For this review, take the finished solid that the model builds, in its own axes (mm). Face numbers are marked on the shaded views. A direction names the side the tool comes from. Coordinates: 2 decimals unless noted, no trailing zeros. Loops run counter-clockwise (first coordinate to the right, second up) from the corner with the lowest first, then second, coordinate; pieces in that order, holes last. Notation, with made-up numbers: (-12, 45.5) -> (13, 45.5) arc R26 ccw to (13, 68.5) -> close; hole circle Ø7 at (20, -38.75). An arc over 180 degrees is marked (long way). Use a Markdown table: item, result.
from build123d import *

# Parameters (mm, degrees)
EXTRUDE_1_DEPTH     = 10
SKETCH_2_R          = 6.5
CUT_EXTRUDE_1_DEPTH = 10
CUT_EXTRUDE_2_DEPTH = 10
FILLET_1_R          = 1
SKETCH_4_R          = 6.5
CUT_EXTRUDE_3_DEPTH = 10


with BuildPart() as part:
    # 草图1 → 凸台-拉伸1 (new body)
    with BuildSketch(Plane.XY):
        with BuildLine():
            Line((200.1875, 14.998828079), (0.21875, 17.498632759))
            ThreePointArc((0.21875, 17.498632759), (-17.5, 0), (0.21875, -17.498632759))
            Line((0.21875, -17.498632759), (200.1875, -14.998828079))
            ThreePointArc((200.1875, -14.998828079), (215, 0), (200.1875, 14.998828079))
        make_face()
    extrude(amount=EXTRUDE_1_DEPTH)

    # 草图2 → 切除-拉伸1 (cut)
    with BuildSketch(Plane.XY.offset(10)):
        Circle(SKETCH_2_R)
    extrude(amount=-CUT_EXTRUDE_1_DEPTH, mode=Mode.SUBTRACT)

    # 草图3 → 切除-拉伸2 (cut)
    with BuildSketch(Plane.XY.offset(10)):
        Polygon((24.289001935, 12.19734043), (85.658139631, 11.430166271), (16.937408094, -6.979422532), align=None)
        Polygon((16.414613885, -12.295777972), (84.346077325, 5.902373893), (91.781134838, -11.353622851), align=None)
        Polygon((106.93275646, -6.06439659), (114.284350301, 13.112366373), (175.653487997, 12.345192214), align=None)
        Polygon((181.776483204, -10.438596909), (106.409962251, -11.380752029), (174.341425691, 6.817399835), align=None)
    extrude(amount=-CUT_EXTRUDE_2_DEPTH, mode=Mode.SUBTRACT)

    # 圆角1
    fillet_1_edges = [part.edges().sort_by_distance(p)[0] for p in [
        (84.346077325, 5.902373893, 5),
        (91.781134838, -11.353622851, 5),
        (16.414613885, -12.295777972, 5),
        (175.653487997, 12.345192214, 5),
        (106.93275646, -6.06439659, 5),
        (114.284350301, 13.112366373, 5),
        (174.341425691, 6.817399835, 5),
        (181.776483204, -10.438596909, 5),
        (106.409962251, -11.380752029, 5),
        (85.658139631, 11.430166271, 5),
        (16.937408094, -6.979422532, 5),
        (24.289001935, 12.19734043, 5),
    ]]
    fillet(fillet_1_edges, radius=FILLET_1_R)

    # 草图4 → 切除-拉伸3 (cut)
    with BuildSketch(Plane.XY.offset(10)):
        with Locations((200, 0)):
            Circle(SKETCH_4_R)
    extrude(amount=-CUT_EXTRUDE_3_DEPTH, mode=Mode.SUBTRACT)


solid = part.part
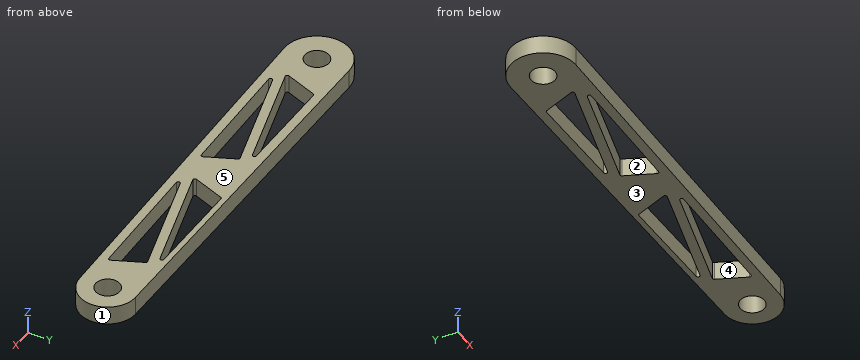
(1) For the marked faces 4 and 5, list the 3-axis set-ups (+Z, -Z, +X, -X, +Y, -Y) from which the entire face can be reached by the end or side of a thin tool; tool diameter is ignored.
Found:
| item | result |
|---|---|
| face 4 | +Z, -Z |
| face 5 | +Z, +X, -X, +Y, -Y |
(2) For pin 1 Ø11.5 at (x, y) = (0, 0) entering from -Z (3 decimals); pin 2 Ø1.5 at (x, z) = (46, 2) entering from +Y; pin 3 Ø2 at (y, z) = (13, 7.5) entering from +X; pin 4 Ø1.5 at (x, z) = (189, 3.5) entering from -Y, all flat-tipped, find the tip position at first contact; note any pin that passes through.
Found:
| item | result |
|---|---|
| pin 1 | passes through |
| pin 2 | stops at y = 16.94 |
| pin 3 | stops at x = 209 |
| pin 4 | stops at y = -15.15 |
(3) Take a section at D-D on x = 97.5. Write out the cut boundary in (y, z), plus the area to 3 significant figures.
Found:
| item | result |
|---|---|
| outline | (-16.28, 0) -> (16.28, 0) -> (16.28, 10) -> (-16.28, 10) -> close |
| area | 326 mm^2 |
(4) Take a section at C-C on y = 0. Write out the cut boundary in (x, z).
Found:
| item | result |
|---|---|
| outline | (-17.5, 0) -> (-6.5, 0) -> (-6.5, 10) -> (-17.5, 10) -> close; (6.5, 0) -> (19.61, 0) -> (19.61, 10) -> (6.5, 10) -> close; (42.99, 0) -> (62.31, 0) -> (62.31, 10) -> (42.99, 10) -> close; (86.89, 0) -> (109.26, 0) -> (109.26, 10) -> (86.89, 10) -> close; (129.57, 0) -> (148.89, 0) -> (148.89, 10) -> (129.57, 10) -> close; (177.28, 0) -> (193.5, 0) -> (193.5, 10) -> (177.28, 10) -> close; (206.5, 0) -> (215, 0) -> (215, 10) -> (206.5, 10) -> close |
(5) Take a section at A-A on x = 196.5. Write out the cut boundary in (y, z).
Found:
| item | result |
|---|---|
| outline | (-15.04, 0) -> (-5.48, 0) -> (-5.48, 10) -> (-15.04, 10) -> close; (5.48, 0) -> (15.04, 0) -> (15.04, 10) -> (5.48, 10) -> close |
(6) For line 1 along Y through (x, z) = (133.5, 2.25); line 2 along Y through (x, z) = (26, 5.25); line 3 along Y through (x, z) = (0, 5.25), list the stretches that pass through material, from the lowest coordinate up.
Found:
| item | result |
|---|---|
| line 1 | y = -15.83 to -11.04, -4.12 to 1.05, 12.87 to 15.83 |
| line 2 | y = -17.18 to -12.18, -9.73 to -4.55, 12.18 to 17.18 |
| line 3 | y = -17.5 to -6.5, 6.5 to 17.5 |
(7) Take a section at B-B on z = 2.5. State how many separate pieces and enclosed holes the cut face has, plus the area to 3 significant figures.
Found:
| item | result |
|---|---|
| separate pieces | 1 |
| enclosed holes | 6 |
| area | 4,610 mm^2 |
(8) Mouldability with a two-part tool opening along X and no side actions: class the marked faces 1, 2 and 3 as pulls with the +X half, pulls with the -X half, needs draft (parallel to the pull), parting line crosses it, or undercut.
Found:
| item | result |
|---|---|
| face 1 | pulls with the +X half |
| face 2 | undercut |
| face 3 | needs draft |
